Part model, mm, in its own coordinate system. A direction names the side the tool comes from. Round coordinates to 2 decimals unless told otherwise and drop trailing zeros. Write each loop counter-clockwise with the first axis right and the second up, starting at its lowest first coordinate (ties: lowest second). Pieces come first, ordered by that corner, then holes. Notation, with made-up numbers: M 1.25,50.5 L 38.25,50.5 A17 ccw 38.25,81.5 Z; hole C 57,42.25 d11. An arc over 180 degrees is marked long. Use one line per item in the form item = value. Start each with the question number.
Item 1: Cut at A-A, the plane z = 18.5. Give the cut face in (x, y).
Item 2: Flat gauge pins, fed straight in: pin 1 Ø6 at (x, z) = (-7.5, 10) entering from +Y; pin 2 Ø11.5 at (x, y) = (28, 23.5) entering from +Z; pin 3 Ø12 at (y, z) = (34.5, 36.5) entering from +X. Where does each tip first touch, or does it go through?
Item 3: Cut at C-C, the plane y = 38.1. Give the cut face in (x, z), then the cut area to 3 significant figures.
Item 4: Cut at B-B, the plane x = 25. Give the cut face in (y, z), then the cut area to 3 significant figures.
Item 5: Mould opens along X. For faces 1 (the face through (58, 5, 21)), 2 (the face through (58.48, 4.01, 35.1)), 3 (the face through (0, 23, 21)) say: +X half, -X half, draft (parallel to the pull), parting line (faces both ways), or undercut.
Item 6: Cut at D-D, the plane x = 57.5. State how many separate pieces and enclosed holes the cut face has, then the cut area to 3 significant figures.
Item 7: Probe L1, parallel to X at y = 1.8, z = 10; L2, parallel to Z at x = 57.5, y = 42.3; L3, parallel to X at y = 34, z = 33. List the from-to ranges inside material, lowest first.
Item 8: Which spindle directions (+Z, -Z, +X, -X, +Y, -Y) get a long thin tool onto all of the face, cutting with end or side? Do faces 4 (the face through (-8.9, 3, 11.4)), 5 (the face through (58.933, 1.479, 31.086)), 6 (the face through (57, 40.8, 21)). Say none if no direction does.
from build123d import *

# Parameters (mm, degrees)
ESQUISSE1_R                                     = 2
ESQUISSE1_R_2                                   = 11
BOSS_EXTRU_1_DEPTH                              = 2
BOSS_EXTRU_2_DEPTH                              = 40
CHAMBRAGE_POUR_VIS_T_TE_CYLINDRIQUE_D           = 3.4
CHAMBRAGE_POUR_VIS_T_TE_CYLINDRIQUE_DEPTH       = 5
CHAMBRAGE_POUR_VIS_T_TE_CYLINDRIQUE_CBORE_D     = 6.5
CHAMBRAGE_POUR_VIS_T_TE_CYLINDRIQUE_CBORE_DEPTH = 2


with BuildPart() as part:
    # Esquisse1 → Boss.-Extru.1 (new body)
    with BuildSketch(Plane.XY):
        Polygon((0, 5), (-15, 5), (-15, 0), (65, 0), (65, 5), (50, 5), (50, 40.8), (65, 40.8), (65, 45.8), (-15, 45.8), (-15, 40.8), (0, 40.8), align=None)
        with Locations((25, 38.1)):
            Circle(ESQUISSE1_R, mode=Mode.SUBTRACT)
        with Locations((11.836413862, 15.3)):
            Circle(ESQUISSE1_R, mode=Mode.SUBTRACT)
        with Locations((38.163586138, 15.3)):
            Circle(ESQUISSE1_R, mode=Mode.SUBTRACT)
        with Locations((25, 22.9)):
            Circle(ESQUISSE1_R_2, mode=Mode.SUBTRACT)
    extrude(amount=BOSS_EXTRU_1_DEPTH)

    # Esquisse3 → Boss.-Extru.2 (add)
    with BuildSketch(Plane.XY.offset(2)):
        with BuildLine():
            Line((-15, 40.8), (0, 40.8))
            Line((0, 40.8), (9.470292352, 34.019270676))
            ThreePointArc((9.470292352, 34.019270676), (25, 42), (40.529707648, 34.019270676))
            Line((40.529707648, 34.019270676), (50, 40.8))
            Line((50, 40.8), (65, 40.8))
            Line((65, 40.8), (65, 45.8))
            Line((65, 45.8), (-15, 45.8))
            Line((-15, 45.8), (-15, 40.8))
        make_face()
        with BuildLine():
            Line((9.470292352, 34.019270676), (0, 40.8))
            Line((0, 40.8), (0, 5))
            Line((0, 5), (9.470292352, 11.780729324))
            ThreePointArc((9.470292352, 11.780729324), (5.9, 22.9), (9.470292352, 34.019270676))
        make_face()
        with BuildLine():
            Line((9.470292352, 11.780729324), (0, 5))
            Line((0, 5), (-15, 5))
            Line((-15, 5), (-15, 0))
            Line((-15, 0), (65, 0))
            Line((65, 0), (65, 5))
            Line((65, 5), (50, 5))
            Line((50, 5), (40.529707648, 11.780729324))
            ThreePointArc((40.529707648, 11.780729324), (25, 3.8), (9.470292352, 11.780729324))
        make_face()
        with BuildLine():
            Line((50, 40.8), (40.529707648, 34.019270676))
            ThreePointArc((40.529707648, 34.019270676), (43.185535682, 28.739203024), (44.1, 22.9))
            ThreePointArc((44.1, 22.9), (43.185535682, 17.060796976), (40.529707648, 11.780729324))
            Line((40.529707648, 11.780729324), (50, 5))
            Line((50, 5), (50, 40.8))
        make_face()
    extrude(amount=BOSS_EXTRU_2_DEPTH)

    # Chambrage pour vis à tête cylindrique à 6 pans creux (ou vis CHC) M31
    with Locations(Plane(origin=(57.5, 5, 32), x_dir=(0, 0, 1), z_dir=(0, 1, 0))):
        with Locations((0, 0), (-22, 0), (-22, -65), (0, -65)):
            chambrage_pour_vis_t_te_cylindrique = CounterBoreHole(CHAMBRAGE_POUR_VIS_T_TE_CYLINDRIQUE_D / 2, CHAMBRAGE_POUR_VIS_T_TE_CYLINDRIQUE_CBORE_D / 2, CHAMBRAGE_POUR_VIS_T_TE_CYLINDRIQUE_CBORE_DEPTH, depth=CHAMBRAGE_POUR_VIS_T_TE_CYLINDRIQUE_DEPTH)

    # Symétrie1: Chambrage pour vis à tête cylindrique à 6 pans creux (ou vis CHC) M31 across plane
    add(chambrage_pour_vis_t_te_cylindrique.mirror(Plane.ZX.offset(22.9)), mode=Mode.SUBTRACT)


solid = part.part
Model answer:
q1.outline = M -15,0 L 65,0 L 65,5 L 50,5 L 50,40.8 L 65,40.8 L 65,45.8 L -15,45.8 L -15,40.8 L 0,40.8 L 0,5 L -15,5 Z; hole C 25,22.9 d38.2
q2.pin_1 = 45.8
q2.pin_2 = through
q2.pin_3 = 50
q3.outline = M 0,0 L 23,0 L 23,2 L 13.43,2 L 13.43,42 L 0,42 Z; M 27,0 L 50,0 L 50,42 L 36.57,42 L 36.57,2 L 27,2 Z
q3.area = 1,170 mm²
q4.outline = M 0,0 L 11.9,0 L 11.9,2 L 3.8,2 L 3.8,42 L 0,42 Z; M 33.9,0 L 36.1,0 L 36.1,2 L 33.9,2 Z; M 40.1,0 L 45.8,0 L 45.8,42 L 42,42 L 42,2 L 40.1,2 Z
q4.area = 344 mm²
q5.face_1 = draft
q5.face_2 = undercut
q5.face_3 = -X half
q6.separate_pieces = 6
q6.enclosed_holes = 0
q6.area = 327 mm²
q7.L1 = -15 to -9.2, -5.8 to 55.8, 59.2 to 65
q7.L2 = 0 to 6.75, 13.25 to 28.75, 35.25 to 42
q7.L3 = 0 to 9.46, 40.54 to 50
q8.face_4 = none
q8.face_5 = +Y, -Y
q8.face_6 = +Z, -Z, +X
